Autodesk Inventor part; units mm, degrees
ref_plane "Work Plane1" through (86, 160, 0) normal (0, 0.9659258, -0.258819) x (-1, 0, 0)
ref_plane "YZ Plane" through (0, 0, 0) normal (1, 0, 0) x (0, 1, 0)
ref_plane "XZ Plane" through (0, 0, 0) normal (0, 1, 0) x (-1, 0, 0)
sketch "Sketch1" plane through (0, 0, 0) normal (0, 0, 1) x (1, 0, 0)
  line L0 (-86, -160) -> (86, -160)
  line L1 (86, -160) -> (86, 160)
  line L2 (86, 160) -> (-86, 160)
  line L3 (-86, 160) -> (-86, -160)
  line L4 (-86, -160) -> (86, 160) construction
  line L5 (86, -160) -> (-86, 160) construction
  point P0 (0, 0)
  dimension "d0" = 320
  dimension "d1" = 172
extrude "Plate1" add sketch "Sketch1" along normal blind 3.048
sketch "Sketch2" plane through (0, 0, 3.048) normal (0, 0, 1) x (1, 0, 0)
  circle A0 centre (-76, 149) radius 3.25
  line L0 (0, 144.4317) -> (0, -177.0748)
  line L1 (-144.6038, 10) -> (151.531, 10)
  circle A1 centre (76, 149) radius 3.25
  circle A2 centre (-76, -129) radius 3.25
  circle A3 centre (76, -129) radius 3.25
  point P0 (0, 0)
  dimension "d3" = 0
  dimension "d4" = 10
  dimension "d5" = 6.5
  dimension "d6" = 76
  dimension "d7" = 139
extrude "Cut1" cut sketch "Sketch2" against normal blind 3.048
sketch "Sketch3" plane through (0, 0, 3.048) normal (0, 0, 1) x (1, 0, 0)
  line L0 (-76, -152.5) -> (-76, -147.5) construction
  line L1 (-78.5, -152.5) -> (-78.5, -147.5)
  line L2 (-73.5, -147.5) -> (-73.5, -152.5)
  arc A0 (-78.5, -152.5) -> (-73.5, -152.5) centre (-76, -152.5) ccw
  arc A1 (-73.5, -147.5) -> (-78.5, -147.5) centre (-76, -147.5) ccw
  line L3 (76, -152.5) -> (76, -147.5) construction
  line L4 (73.5, -152.5) -> (73.5, -147.5)
  line L5 (78.5, -147.5) -> (78.5, -152.5)
  arc A2 (73.5, -152.5) -> (78.5, -152.5) centre (76, -152.5) ccw
  arc A3 (78.5, -147.5) -> (73.5, -147.5) centre (76, -147.5) ccw
  line L6 (-23.5, 120) -> (-28.5, 120) construction
  line L7 (-23.5, 122.5) -> (-28.5, 122.5) construction
  line L8 (-28.5, 117.5) -> (-23.5, 117.5) construction
  arc A4 (-23.5, 117.5) -> (-23.5, 122.5) centre (-23.5, 120) ccw construction
  arc A5 (-28.5, 122.5) -> (-28.5, 117.5) centre (-28.5, 120) ccw construction
  line L9 (76, 17.5) -> (76, 22.5) construction
  line L10 (78.5, 17.5) -> (78.5, 22.5)
  line L11 (73.5, 22.5) -> (73.5, 17.5)
  arc A6 (73.5, 17.5) -> (78.5, 17.5) centre (76, 17.5) ccw
  arc A7 (78.5, 22.5) -> (73.5, 22.5) centre (76, 22.5) ccw
  line L12 (86, -160) -> (-86, -160)
  line L13 (-86, 160) -> (86, 160)
  line L14 (-86, -160) -> (-86, 160)
  line L15 (-76, 17.5) -> (-76, 22.5) construction
  line L16 (-78.5, 17.5) -> (-78.5, 22.5)
  line L17 (-73.5, 22.5) -> (-73.5, 17.5)
  arc A8 (-78.5, 17.5) -> (-73.5, 17.5) centre (-76, 17.5) ccw
  arc A9 (-73.5, 22.5) -> (-78.5, 22.5) centre (-76, 22.5) ccw
  line L18 (86, 160) -> (86, -160)
  point P0 (0, 0)
  point P1 (-76, -150)
  point P2 (76, -150)
  point P3 (-26, 120)
  point P4 (76, 20)
  point P5 (-76, 20)
  dimension "d12" = 10
  dimension "d13" = 10
  dimension "d14" = 170
  dimension "d16" = 40
  dimension "d17" = 0
  dimension "d18" = 60
  dimension "d19" = 170
  dimension "d20" = 0
  dimension "d21" = 5
  dimension "d22" = 5
  dimension "d23" = 5
  dimension "d24" = 5
  dimension "d25" = 5
  dimension "d26" = 2.5
  dimension "d27" = 2.5
  dimension "d28" = 2.5
  dimension "d29" = 2.5
  dimension "d30" = 2.5
  dimension "d33" = 10
  dimension "d34" = 10
extrude "Cut2" cut sketch "Sketch3" against normal blind 3.048 contours L1 A1 L2 A0 | L4 A3 L5 A2 | A6 L11 A7 L10 | L16 A9 L17 A8
ref_plane "Work Plane1" through (86, 160, 0) normal (0, 0.9659258, -0.258819) x (-1, 0, 0)
fillet "Fillet1" radius 10 2 edges at (-86, -160, 1.524) (86, -160, 1.524)
sketch "Sketch7" plane through (0, 0, 3.048) normal (0, 0, 1) x (1, 0, 0)
  line L0 (86, 160) -> (-86, 160)
  line L1 (-86, 160) -> (86, 160)
  line L2 (86, 160) -> (86, 180)
  line L3 (86, 180) -> (-86, 180)
  line L4 (-86, 180) -> (-86, 160)
  point P0 (0, 0)
  dimension "d50" = 20
sheet face with bend "Face4" sketch "Sketch7" thickness 3.048 toward (0, 0, -1) bend radius 3.048
bend "Bend3"
sketch "Sketch8" plane through (0, 0, 3.048) normal (0, 0, 1) x (1, 0, 0)
  line L0 (0, 167.5) -> (0, 172.5) construction
  line L1 (2.5, 167.5) -> (2.5, 172.5)
  line L2 (-2.5, 172.5) -> (-2.5, 167.5)
  arc A0 (-2.5, 167.5) -> (2.5, 167.5) centre (0, 167.5) ccw
  arc A1 (2.5, 172.5) -> (-2.5, 172.5) centre (0, 172.5) ccw
  line L3 (86, 180) -> (-86, 180)
  line L4 (86, 180) -> (86, -150)
  line L5 (-86, 180) -> (-86, -150)
  point P0 (0, 0)
  point P1 (0, 170)
  dimension "d56" = 2.5
  dimension "d57" = 5
  dimension "d58" = 10
  dimension "d59" = 172
  dimension "d60" = 86
extrude "Cut3" cut sketch "Sketch8" against normal blind 3.048
fillet "Corner Round1" radius 10 2 edges at (86, 180, 1.524) (-86, 180, 1.524)
chamfer "Chamfer1" distance 0.75 angle 45 8 edges at (0, -160, 3.048) (-83.0711, -157.0711, 3.048) (-86, 10, 3.048) (-83.0711, 177.0711, 3.048) (0, 180, 3.048) (83.0711, 177.0711, 3.048) (86, 10, 3.048) (83.0711, -157.0711, 3.048)
equation "\"d22\" = d21"
equation "\"d23\" = d21"
equation "\"d24\" = d21"
equation "\"d25\" = d21"
equation "\"d27\" = d26"
equation "\"d28\" = d26"
equation "\"d29\" = d28"
equation "\"d30\" = d28"
equation "\"BendRadius\" = Thickness"
equation "\"BendReliefWidth\" = Thickness"
equation "\"BendReliefDepth\" = 0.5 * Thickness"
equation "\"CornerReliefSize\" = 4 * Thickness"
equation "\"MinimumRemnant\" = 2 * Thickness"
equation "\"TransitionRadius\" = BendRadius"
equation "\"JacobiRadiusSize\" = BendRadius"
equation "\"GapSize\" = Thickness"
properties part number "CCU_Fix"
Here's how the part is built. I have some questions about the finished solid (model axes, mm). Give positions to 0.01 mm unless a question says otherwise; leave off trailing zeros. Loops run counter-clockwise (first coordinate to the right, second up) from the corner with the lowest first, then second, coordinate; pieces in that order, holes last. Notation, with made-up numbers: M 37.25,28.5 L 49.25,28.5 A30 cw 49.25,52.5 Z; hole C 30,35.25 d8. An arc over 180 degrees is marked long. Return JSON: item names as keys, results as strings.
Item 1: Please list where these lines run through material, in increasing order: line 1 (Y direction, x = -76, z = 0.9); line 2 (X direction, y = -129, z = 1.25); line 3 (Y direction, x = -76, z = 2.35).
A:
{"line 1": "y = -160 to -155, -145 to -132.25, -125.75 to 15, 25 to 145.75, 152.25 to 180", "line 2": "x = -86 to -79.25, -72.75 to 72.75, 79.25 to 86", "line 3": "y = -159.95 to -155, -145 to -132.25, -125.75 to 15, 25 to 145.75, 152.25 to 179.95"}
Item 2: Imagine slicing it at A-A on y = -129. List the corners of the cut face in (x, z) for me, then the cut area to 3 significant figures.
A:
{"outline": "M -86,0 L -79.25,0 L -79.25,3.05 L -85.25,3.05 L -86,2.3 Z; M -72.75,0 L 72.75,0 L 72.75,3.05 L -72.75,3.05 Z; M 79.25,0 L 86,0 L 86,2.3 L 85.25,3.05 L 79.25,3.05 Z", "area": "484 mm^2"}
Item 3: Thinking about a two-plate mould opening in Y: for faces 1 (the cylindrical face through (-78.579, -130.978, 1.545)), 2 (the cylindrical face through (-78.395, 151.197, 1.545)), 3 (the conical face through (-82.705, 176.56, 2.918)), 4 (the conical face through (82.705, -156.56, 2.918)), which applies, released by +Y, released by -Y, zero draft, split by the parting line, or undercut?
A:
{"face 1": "undercut", "face 2": "undercut", "face 3": "released by +Y", "face 4": "released by -Y"}
Item 4: I'm going to push a flat-ended pin straight in: pin 1 Ø1.5 at (y, z) = (20, 2.5) entering from -X. Where does the tip first touch, or does it pass through?
A:
{"pin 1": "stops at x = -86"}
